The model under review builds one solid part; all positions refer to its coordinate system, in mm. Face numbers are marked on the shaded views. A direction names the side the tool comes from. Round coordinates to 2 decimals unless told otherwise and drop trailing zeros. Write each loop counter-clockwise with the first axis right and the second up, starting at its lowest first coordinate (ties: lowest second). Pieces come first, ordered by that corner, then holes. Notation, with made-up numbers: (-9, 45) -> (35, 45) arc R14 ccw to (35, 64) -> close; hole circle Ø8 at (6, 3). An arc over 180 degrees is marked (long way). Answer as a JSON object with one key per item and string values. Group by question number.
1) We need section C-C, the plane z = 8.5. Write out the cut boundary in (x, y).
2) We need section B-B, the plane y = 9. Write out the cut boundary in (x, z), then the cut area to 3 significant figures.
3) Machinability: for the marked faces 1 and 2, which of the approach directions +Z, -Z, +X, -X, +Y, -Y give a long, thin tool a straight path to every point of the face, cutting with its end or side? Answer none if there is none.
4) We need section A-A, the plane x = -55.5. Write out the cut boundary in (y, z), then the cut area to 3 significant figures.
5) To check wall thickness, follow probe 1 along Y at (x, z) = (-42, 5); probe 2 along X at (y, z) = (10.75, 7.5); probe 3 along Z at (x, y) = (-48.5, 0.25). State the ranges of each line that lie inside material, in increasing order. Write a range as [from, to].
6) Mouldability with a two-part tool opening along Y and no side actions: class the marked faces 3, 4 and 5 as pulls with the +Y half, pulls with the -Y half, needs draft (parallel to the pull), parting line crosses it, or undercut.
7) Insertion check: pin 1 Ø8 at (x, y) = (-59.5, 8.5) entering from -Z; pin 2 Ø0.6 at (y, z) = (16, -1) entering from +X; pin 3 Ø0.6 at (x, y) = (-37.5, 0.5) entering from -Z. Each pin has a flat end and moves straight along its axis. Give the tip position at first contact, or say it passes through.
from build123d import *

# Parameters (mm, degrees)
ESQUISSE1_W             = 36.8
ESQUISSE1_H             = 20
ESQUISSE1_W_2           = 35.8
ESQUISSE1_H_2           = 19
BASE_EXTRUSION_DEPTH    = 14
ESQUISSE2_W             = 36.8
ESQUISSE2_H             = 20
BOSS_EXTRU_1_DEPTH      = 1
ENL_V_MAT_EXTRU_1_DEPTH = 43.872204303
ESQUISSE4_W             = 1
ESQUISSE4_H             = 0.5
BOSS_EXTRU_2_DEPTH      = 2


with BuildPart() as part:
    # Esquisse1 → Base-Extrusion (new body)
    with BuildSketch(Plane.XY):
        with Locations((-55.64228109, 6.086823856)):
            Rectangle(ESQUISSE1_W, ESQUISSE1_H)
        with Locations((-55.64228109, 6.086823856)):
            Rectangle(ESQUISSE1_W_2, ESQUISSE1_H_2, mode=Mode.SUBTRACT)
    extrude(amount=BASE_EXTRUSION_DEPTH)

    # Esquisse2 → Boss.-Extru.1 (add)
    with BuildSketch(Plane.XY.offset(14)):
        with Locations((-55.64228109, 6.086823856)):
            Rectangle(ESQUISSE2_W, ESQUISSE2_H)
    extrude(amount=BOSS_EXTRU_1_DEPTH)

    # Esquisse3 → Enlèv. mat.-Extru.1 (cut, through all)
    with BuildSketch(Plane(origin=(-37.24228109, 0, 0), x_dir=(0, 0, -1), z_dir=(1, 0, 0))):
        with BuildLine():
            Line((0.67598994, 7.836823856), (0.67598994, 4.336823856))
            Line((0.67598994, 4.336823856), (-3.3, 4.336823856))
            ThreePointArc((-3.3, 4.336823856), (-5.05, 6.086823856), (-3.3, 7.836823856))
            Line((-3.3, 7.836823856), (0.67598994, 7.836823856))
        make_face()
    extrude(amount=-ENL_V_MAT_EXTRU_1_DEPTH, mode=Mode.SUBTRACT)

    # Esquisse4 → Boss.-Extru.2 (add)
    with BuildSketch(Plane(origin=(0, 0, 0), x_dir=(-1, 0, 0), z_dir=(0, 0, -1))):
        with Locations((38.24228109, 15.836823856)):
            Rectangle(ESQUISSE4_W, ESQUISSE4_H)
        with Locations((73.04228109, 15.836823856)):
            Rectangle(ESQUISSE4_W, ESQUISSE4_H)
        with Locations((73.04228109, -3.663176144)):
            Rectangle(ESQUISSE4_W, ESQUISSE4_H)
        with Locations((38.24228109, -3.663176144)):
            Rectangle(ESQUISSE4_W, ESQUISSE4_H)
    extrude(amount=BOSS_EXTRU_2_DEPTH)


solid = part.part
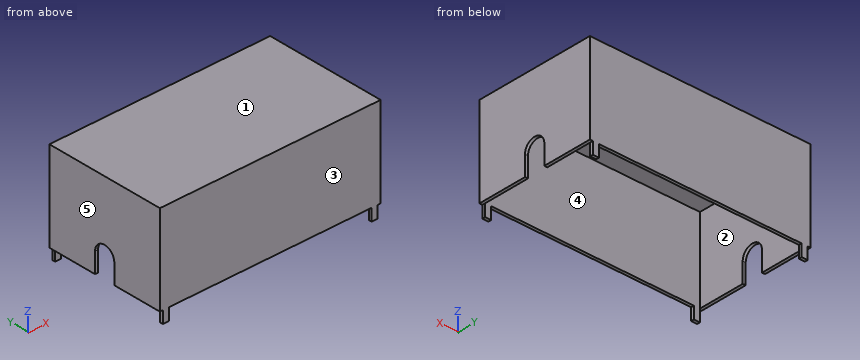
Here are the results:
{
 "1": {"outline": "(-74.04, -3.91) -> (-37.24, -3.91) -> (-37.24, 16.09) -> (-74.04, 16.09) -> close; hole (-73.54, -3.41) -> (-37.74, -3.41) -> (-37.74, 15.59) -> (-73.54, 15.59) -> close"},
 "2": {"outline": "(-74.04, 0) -> (-73.54, 0) -> (-73.54, 14) -> (-37.74, 14) -> (-37.74, 0) -> (-37.24, 0) -> (-37.24, 15) -> (-74.04, 15) -> close", "area": "50.8 mm^2"},
 "3": {"face 1": "+Z, +X, -X, +Y, -Y", "face 2": "-Z"},
 "4": {"outline": "(-3.91, 0) -> (-3.41, 0) -> (-3.41, 14) -> (15.59, 14) -> (15.59, 0) -> (16.09, 0) -> (16.09, 15) -> (-3.91, 15) -> close", "area": "34.0 mm^2"},
 "5": {"probe 1": "y = [-3.91, -3.41], [15.59, 16.09]", "probe 2": "x = [-74.04, -73.54], [-37.74, -37.24]", "probe 3": "z = [14, 15]"},
 "6": {"face 3": "pulls with the -Y half", "face 4": "undercut", "face 5": "needs draft"},
 "7": {"pin 1": "stops at z = 14", "pin 2": "stops at x = -37.74", "pin 3": "stops at z = 0"}
}
